Design review of the part shown in the three views and the two pictorial views. Dimensions are in mm from the part's minimum x, y and z. Round coordinates to 2 decimals unless told otherwise and drop trailing zeros. Write each loop counter-clockwise with the first axis right and the second up, starting at its lowest first coordinate (ties: lowest second). Pieces come first, ordered by that corner, then holes. Notation, with made-up numbers: (4.5, 51) - (50.5, 51) arc R12 ccw to (50.5, 72) - close; hole circle Ø6 at (-18.5, 72). An arc over 180 degrees is marked (long way). Use one line per item in the form item = value.
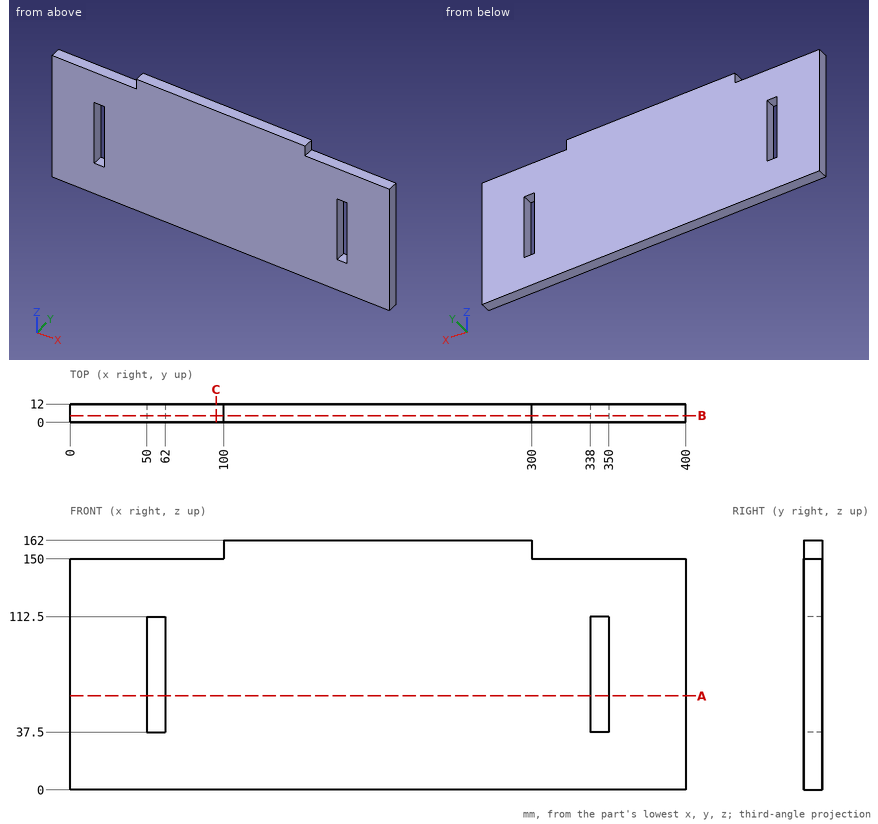
(1) Add section B-B on y = 4.5. Write out the cut boundary in (x, z).
Geometry results:
outline = (0, 0) - (400, 0) - (400, 150) - (300, 150) - (300, 162) - (100, 162) - (100, 150) - (0, 150) - close; hole (50, 37.5) - (62, 37.5) - (62, 112.5) - (50, 112.5) - close; hole (338, 37.5) - (350, 37.5) - (350, 112.5) - (338, 112.5) - close
(2) Add section C-C on x = 95. Write out the cut boundary in (y, z), then the cut area to 3 significant figures.
Geometry results:
outline = (0, 0) - (12, 0) - (12, 150) - (0, 150) - close
area = 1,800 mm2
(3) To check wall thickness, follow L1, parallel to X at y = 4.75, z = 44.5; L2, parallel to Z at x = 349.5, y = 2.5; L3, parallel to Z at x = 351, y = 6.5. State the ranges of each line that lie inside material, in increasing order.
Geometry results:
L1 = 0 to 50, 62 to 338, 350 to 400
L2 = 0 to 37.5, 112.5 to 150
L3 = 0 to 150
(4) Insertion check: P1, Ø6, axis at x = 150, y = 5.5, coming from the -Z side; P2, Ø6, axis at x = 53, y = 8.5, coming from the +Z side; P3, Ø3.5, axis at y = 5.5, z = 155.5, coming from the -X side. Each pin has a flat end and moves straight along its axis. Give the tip position at first contact, or say it passes through.
Geometry results:
P1 = 0
P2 = 150
P3 = 100
(5) Add section A-A on z = 61. Write out the cut boundary in (x, y), then the cut area to 3 significant figures.
Geometry results:
outline = (0, 0) - (50, 0) - (50, 12) - (0, 12) - close; (62, 0) - (338, 0) - (338, 12) - (62, 12) - close; (350, 0) - (400, 0) - (400, 12) - (350, 12) - close
area = 4,510 mm2
